Input: dimensioned drawing with shaded views. Units: mm. Origin: part minimum x, y, z. Give positions to 0.01 mm unless a question says otherwise; leave off trailing zeros. Order: outer loops, then holes, each group sorted by start corner. A loop starts at its lowest first (then second) coordinate and runs counter-clockwise, first axis right, second up. Notation, with made-up numbers: (71, 16.25) - (113, 16.25) arc R16 ccw to (113, 35.25) - close; hole circle Ø8 at (33, -9.5). An arc over 180 degrees is marked (long way). Use a Markdown table: item, result.
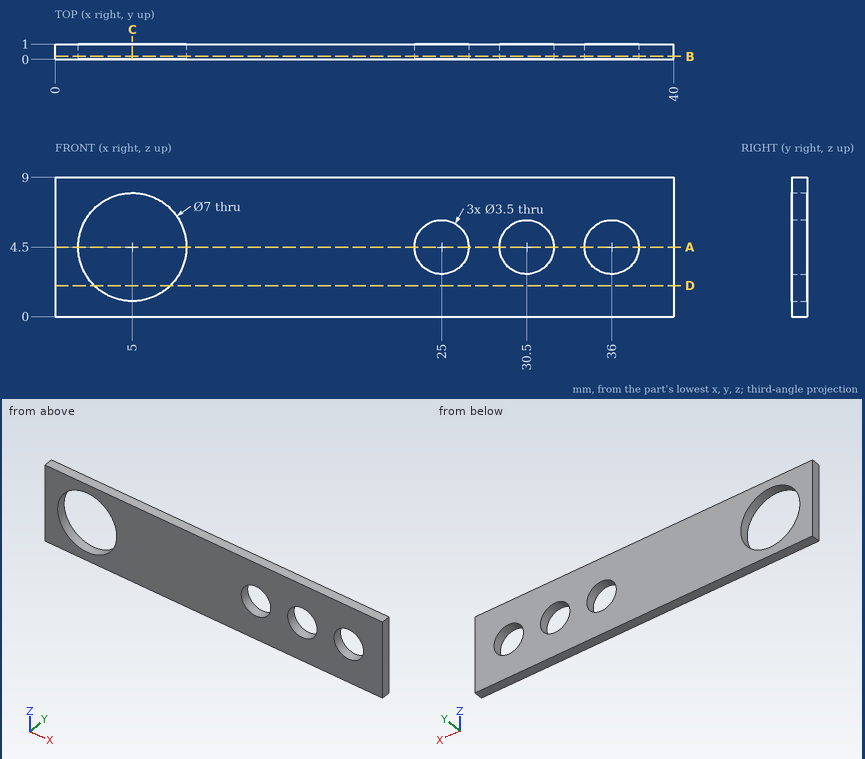
1. Section query D-D (z = 2). Return loops of the section in (x, y), then the cut area to 3 significant figures.
Response:
| item | result |
|---|---|
| outline | (0, 0) - (2.55, 0) - (2.55, 1) - (0, 1) - close; (7.45, 0) - (40, 0) - (40, 1) - (7.45, 1) - close |
| area | 35.1 mm^2 |
2. Material intervals for line 1 along X through (y, z) = (0.4, 4.5); line 2 along Z through (x, y) = (5, 0.55); line 3 along Z through (x, y) = (36, 0.85), sorted ascending.
Response:
| item | result |
|---|---|
| line 1 | x = 0 to 1.5, 8.5 to 23.25, 26.75 to 28.75, 32.25 to 34.25, 37.75 to 40 |
| line 2 | z = 0 to 1, 8 to 9 |
| line 3 | z = 0 to 2.75, 6.25 to 9 |
3. Section query C-C (x = 5). Return loops of the section in (y, z).
Response:
| item | result |
|---|---|
| outline | (0, 0) - (1, 0) - (1, 1) - (0, 1) - close; (0, 8) - (1, 8) - (1, 9) - (0, 9) - close |
4. Section query A-A (z = 4.5). Return loops of the section in (x, y).
Response:
| item | result |
|---|---|
| outline | (0, 0) - (1.5, 0) - (1.5, 1) - (0, 1) - close; (8.5, 0) - (23.25, 0) - (23.25, 1) - (8.5, 1) - close; (26.75, 0) - (28.75, 0) - (28.75, 1) - (26.75, 1) - close; (32.25, 0) - (34.25, 0) - (34.25, 1) - (32.25, 1) - close; (37.75, 0) - (40, 0) - (40, 1) - (37.75, 1) - close |
5. Section query B-B (y = 0.2). Return loops of the section in (x, z), then the cut area to 3 significant figures.
Response:
| item | result |
|---|---|
| outline | (0, 0) - (40, 0) - (40, 9) - (0, 9) - close; hole circle Ø7 at (5, 4.5); hole circle Ø3.5 at (25, 4.5); hole circle Ø3.5 at (30.5, 4.5); hole circle Ø3.5 at (36, 4.5) |
| area | 293 mm^2 |
